Source: CAD feature listing. Evaluate the final solid. Frame: model axes, mm. A direction names the side the tool comes from. Coordinates: 2 decimals unless noted, no trailing zeros. Order: outer loops, then holes, each group sorted by start corner. A loop starts at its lowest first (then second) coordinate and runs counter-clockwise, first axis right, second up.
```python
from build123d import *

# Parameters (mm, degrees)
F0_W        = 100
F0_H        = 50
F1_DEPTH    = 80
F2_T        = -5
F3_R        = 10
F4_DEPTH    = 50
F5_T        = 2.5
F5_T3_DEPTH = 80
F5_T5_DEPTH = 45
F5_T7_DEPTH = 95


# Not quite as in the source:
# - a shell that OpenCascade refuses in one call is made with other operations: the cavity is built on its own and cut out


with BuildPart() as f1:
    # F0 (on Front) → F1 (new body)
    with BuildSketch(Plane.XZ):
        Rectangle(F0_W, F0_H)
    extrude(amount=F1_DEPTH)

    # F2
    f2_openings = [f1.faces().sort_by_distance(p)[0] for p in [
        (0, -80, 0),
    ]]
    offset(amount=F2_T, openings=f2_openings)

    # F3 (on face) → F4 (join)
    with BuildSketch(Plane(origin=(0, 0, 0), x_dir=(-1, 0, 0), z_dir=(0, 1, 0))):
        Circle(F3_R)
    extrude(amount=-F4_DEPTH)

    # F5: shell of thickness 2.5, made by hand


with BuildPart() as f5_core1:
    # F5_t2: copy of F1
    add(f1.part)

    # the walls: a layer under each face that stays
    f5_faces = [f5_core1.faces().sort_by_distance(p)[0] for p in [
        (-50, -40, 0),
        (0, -40, 25),
        (0, -40, -25),
        (0, 0, 0),
        (-42.8571428571, -80, -21.4285714286),
        (50, -40, 0),
        (-45, -42.5, 0),
        (0, -42.5, 20),
        (45, -42.5, 0),
        (0, -42.5, -20),
        (-30, -5, -13.3333333333),
        (10, -27.5, 0),
    ]]
    thicken(f5_faces, amount=-F5_T, mode=Mode.SUBTRACT)

    # F5_s4 → F5_t3 (cut)
    with BuildSketch(Plane.XZ.offset(2.5)):
        Polygon((-44.975, -19.975), (-47.5, -20), (-47.5, -22.5), (-45, -22.5), align=None)
        Polygon((-44.975, 19.975), (-47.5, 20), (-47.5, 22.5), (-45, 22.5), align=None)
        Polygon((44.975, 19.975), (45, 22.5), (47.5, 22.5), (47.5, 20), align=None)
        Polygon((44.975, -19.975), (47.5, -20), (47.5, -22.5), (45, -22.5), align=None)
    extrude(amount=F5_T3_DEPTH, mode=Mode.SUBTRACT)

    # F5_s6 → F5_t5 (cut)
    with BuildSketch(Plane.XY.offset(-22.5)):
        Polygon((-44.975, -5.025), (-47.5, -5), (-47.5, -2.5), (-45, -2.5), align=None)
        Polygon((44.975, -5.025), (47.5, -5), (47.5, -2.5), (45, -2.5), align=None)
    extrude(amount=F5_T5_DEPTH, mode=Mode.SUBTRACT)

    # F5_s8 → F5_t7 (cut)
    with BuildSketch(Plane.YZ.offset(-47.5)):
        Polygon((-5.025, 19.975), (-5, 22.5), (-2.5, 22.5), (-2.5, 20), align=None)
        Polygon((-5.025, -19.975), (-5, -22.5), (-2.5, -22.5), (-2.5, -20), align=None)
    extrude(amount=F5_T7_DEPTH, mode=Mode.SUBTRACT)

    # F5_s9 → F5_t10 (revolve, cut)
    with BuildSketch(Plane.XY):
        Polygon((-10.025, -5.025), (-10, -2.5), (-7.5, -2.5), (-7.5, -5), align=None)
    revolve(axis=Axis((0, -5, 0), (0, 1, 0)), mode=Mode.SUBTRACT)


with BuildPart() as f1_1:
    add(f1.part)

    # what is left inside the walls is the cavity
    f5_cavity = [f5_core1.part.solids().sort_by_distance(p)[0] for p in [
        (7.475, -18.333333, 0),
    ]]
    add(f5_cavity, mode=Mode.SUBTRACT)


solid = f1_1.part
```
1. Section query D-D, the plane y = -61.5. Output: boundary loops of the cut face in (x, z), plus the area to 3 significant figures.
2. Draft query along X for faces 3 (the flat face through (-1, -42, 20)), 4 (the flat face through (-1, -39, 25)), 5 (the flat face through (50, -39, 0)). Return one class per face: +X half, -X half, draft (parallel to the pull), parting line (faces both ways), or undercut.
3. Section query A-A, the plane y = -12.5. Output: boundary loops of the cut face in (x, z).
4. Contact query for flat-ended pins moving along their axis: P1, Ø10, axis at x = -1.5, z = 0, coming from the -Y side; P2, Ø4, axis at x = 11, z = -3.5, coming from the -Y side. Output: stop coordinate, or through.
5. Access query for faces 1 (the flat face through (-1, -39, -25)), 2 (the cylindrical face through (2.17, -27.18, -9.76)). Directions: +Z, -Z, +X, -X, +Y, -Y. A direction counts if a zero-diameter tool reaches every point of the face in a straight line with its end or side. Return the directions, or none.
6. Material intervals for line 1 along Z through (x, y) = (0, -15); line 2 along Z through (x, y) = (-28.5, -31); line 3 along X through (y, z) = (-44, -2), sorted ascending.
7. Section query C-C, the plane z = -14.5. Output: boundary loops of the cut face in (x, y).
8. Section query B-B, the plane x = -39. Output: boundary loops of the cut face in (y, z), plus the area to 3 significant figures.
Answer key:
1. outline: (-50, -25) - (50, -25) - (50, 25) - (-50, 25) - close; hole (-45, -20) - (45, -20) - (45, 20) - (-45, 20) - close
1. area: 1,400 mm2
2. face 3: undercut
2. face 4: draft
2. face 5: +X half
3. outline: (-50, -25) - (50, -25) - (50, 25) - (-50, 25) - close; circle Ø20 at (0, 0); hole (-45, -20) - (45, -20) - (45, 20) - (-45, 20) - close; hole circle Ø15 at (0, 0)
4. P1: stops at y = -2.5
4. P2: stops at y = -50
5. face 1: -Z, +X, -X, +Y, -Y
5. face 2: -Y
6. line 1: z = -25 to -20, -10 to -7.5, 7.5 to 10, 20 to 25
6. line 2: z = -25 to -20, 20 to 25
6. line 3: x = -50 to -45, -9.8 to -7.23, 7.23 to 9.8, 45 to 50
7. outline: (-50, -80) - (-45, -80) - (-45, -5) - (45, -5) - (45, -80) - (50, -80) - (50, 0) - (-50, 0) - close
8. outline: (-80, -25) - (0, -25) - (0, 25) - (-80, 25) - (-80, 20) - (-5, 20) - (-5, -20) - (-80, -20) - close
8. area: 1,000 mm2
